```python
from build123d import *

# Parameters (mm, degrees)
SKETCH1_R           = 14.75
BOSS_EXTRUDE1_DEPTH = 8
SKETCH2_R           = 18.9
BOSS_EXTRUDE2_DEPTH = 4
THREAD1_PITCH       = 3.5
THREAD1_FROM        = 3.5
CHAMFER2_SIZE       = 1
SKETCH3_R           = 2
CUT_EXTRUDE1_DEPTH  = 1


with BuildPart() as part:
    # Sketch1 → Boss-Extrude1 (new body)
    with BuildSketch(Plane(origin=(0, 0, 0), x_dir=(1, 0, 0), z_dir=(0, 1, 0))):
        with Locations(Location((0, 0, 0), (0, 0, 270))):
            Circle(SKETCH1_R)
    extrude(amount=BOSS_EXTRUDE1_DEPTH)

    # Sketch2 → Boss-Extrude2 (add)
    with BuildSketch(Plane(origin=(0, 8, 0), x_dir=(1, 0, 0), z_dir=(0, 1, 0))):
        with Locations(Location((-0.005064595, -0.031492848, 0), (0, 0, 270))):
            Circle(SKETCH2_R)
    extrude(amount=BOSS_EXTRUDE2_DEPTH)

    # Thread1: arcs per turn and ends read off the stored shape
    # Thread1: the profile of Thread Profile1 profile screwed along a right-hand helix through 3.285714 turns, 12 arcs to a turn; built about Z, then put on its axis
    thread1_z = Axis((0, 0, 0), (0, 0, 1))
    thread1_corners = [(14.7503, 0, -0.000173205), (14.7503, 0, 3.062673196), (12.855569438, 0, 1.968749995), (12.855569438, 0, 1.093749995)]
    with BuildLine(mode=Mode.PRIVATE) as thread1_profile:
        Line(thread1_corners[0], thread1_corners[1])
        Line(thread1_corners[1], thread1_corners[2])
        Line(thread1_corners[2], thread1_corners[3])
        Line(thread1_corners[3], thread1_corners[0])
    thread1_cap = Face(thread1_profile.wire())
    thread1_turn_angles = [0, 15, 30, 45, 60, 75, 90, 105, 120, 135, 150, 165, 180, 195, 210, 225, 240, 255, 270, 285, 300, 315, 330, 345, 360]
    thread1_turn_weights = [1, 0.9659258262890683, 1, 0.9659258262890683, 1, 0.9659258262890683, 1, 0.9659258262890683, 1, 0.9659258262890683, 1, 0.9659258262890683, 1, 0.9659258262890683, 1, 0.9659258262890683, 1, 0.9659258262890683, 1, 0.9659258262890683, 1, 0.9659258262890683, 1, 0.9659258262890683, 1]
    thread1_turn_rails = [Edge.make_bspline([Vector(p[0], p[1], 0).rotate(thread1_z, thread1_turn_angles[k]) / thread1_turn_weights[k] + Vector(0, 0, p[2] + THREAD1_PITCH * thread1_turn_angles[k] / 360) for k in range(25)], [0, 0, 0, 1, 1, 2, 2, 3, 3, 4, 4, 5, 5, 6, 6, 7, 7, 8, 8, 9, 9, 10, 10, 11, 11, 12, 12, 12], 2, thread1_turn_weights) for p in thread1_corners]
    thread1_turn_sides = [Face.make_surface_from_curves(thread1_turn_rails[p[0]], thread1_turn_rails[p[1]]) for p in [(0, 1), (1, 2), (2, 3), (3, 0)]]
    thread1_last_angles = [1080, 1095, 1110, 1125, 1140, 1155, 1170, 1176.428571429, 1182.857142857]
    thread1_last_weights = [1, 0.9659258262890683, 1, 0.9659258262890683, 1, 0.9659258262890683, 1, 0.9937122098932428, 1]
    thread1_last_rails = [Edge.make_bspline([Vector(p[0], p[1], 0).rotate(thread1_z, thread1_last_angles[k]) / thread1_last_weights[k] + Vector(0, 0, p[2] + THREAD1_PITCH * thread1_last_angles[k] / 360) for k in range(9)], [0, 0, 0, 1, 1, 2, 2, 3, 3, 4, 4, 4], 2, thread1_last_weights) for p in thread1_corners]
    thread1_last_sides = [Face.make_surface_from_curves(thread1_last_rails[p[0]], thread1_last_rails[p[1]]) for p in [(0, 1), (1, 2), (2, 3), (3, 0)]]
    thread1 = Plane(origin=(0, 11.5, 0), x_dir=(-1, 0, 0), z_dir=(0, -1, 0)) * split(Solid(Shell([*[p.moved(Location((0, 0, THREAD1_PITCH * i))) for i in range(3) for p in thread1_turn_sides], *thread1_last_sides, thread1_cap, thread1_cap.rotate(thread1_z, 1182.857142857).moved(Location((0, 0, THREAD1_PITCH * 1182.857142857 / 360)))])), bisect_by=Plane.XY.offset(THREAD1_FROM), keep=Keep.TOP, mode=Mode.PRIVATE)
    add(thread1, mode=Mode.SUBTRACT)

    # Chamfer2
    chamfer2_edges = [part.edges().sort_by_distance(p)[0] for p in [
        (-0.005064595, 12, -18.868507152),
    ]]
    chamfer(chamfer2_edges, length=CHAMFER2_SIZE)

    # Sketch3 → Cut-Extrude1 (cut)
    with BuildSketch(Plane.XZ):
        with Locations(Location((0, 0, 0), (0, 0, 270))):
            Circle(SKETCH3_R)
    extrude(amount=-CUT_EXTRUDE1_DEPTH, mode=Mode.SUBTRACT)


solid = part.part
```
Model file for the job. Use its own axes, mm. A direction names the side the tool comes from. Round coordinates to 2 decimals unless told otherwise and drop trailing zeros. Write each loop counter-clockwise with the first axis right and the second up, starting at its lowest first coordinate (ties: lowest second). Pieces come first, ordered by that corner, then holes. Notation, with made-up numbers: (12.25, 26) - (34.25, 26) arc R13 ccw to (34.25, 50) - close; hole circle Ø8 at (36.25, 63). An arc over 180 degrees is marked (long way). Use CSV: the item, a comma, the result in double quotes. Start each with the question number.
Item 1: Two-plate mould, pull along Z, no slides. Class faces 3 (the face through (0, 1, 0)), 4 (the face through (0, 12, 0)), 5 (the face through (5.67, 9.48, 18.06)), 6 (the face through (-1.952, 0.493, 0.434)): released by +Z, released by -Z, zero draft, split by the parting line, or undercut.
Item 2: Drill centre lines: L1, parallel to Y at x = 13.5, z = 2; L2, parallel to Y at x = 7.5, z = 13.5; L3, parallel to X at y = 10.25, z = -14.5. Where is each one in solid material? Low to high. Write a range as [from, to].
Item 3: Band-saw the part on A-A (y = 9.25). Write the cut outline in (x, z).
Item 4: Tool access for faces 1 (the face through (-2, 0, -1)), 2 (the face through (4.5, 8, 12.4)): list every direction of +Z, -Z, +X, -X, +Y, -Y with a clear straight run to the whole face (end or side of a thin tool).
Item 5: Pin check, flat tips, straight feed: P1, Ø6, axis at y = 7, z = -10.5, coming from the -X side; P2, Ø6, axis at x = -14, y = 9.5, coming from the -Z side; P3, Ø1, axis at x = -13.5, y = 4.5, coming from the -Z side. Stop position of each tip, or through.
Checked values:
1,face 3,"undercut"
1,face 4,"zero draft"
1,face 5,"split by the parting line"
1,face 6,"undercut"
2,L1,"y = [0, 0.24], [2.03, 3.74], [5.53, 7.24], [8, 12]"
2,L2,"y = [8, 12]"
2,L3,"x = [-12.09, 12.08]"
3,outline,"circle Ø37.8 at (-0.01, 0.03)"
4,face 1,"+Z, -Z, +X, -X, -Y"
4,face 2,"none"
5,P1,"stops at x = -17.26"
5,P2,"stops at z = -15.34"
5,P3,"stops at z = -6.97"
